Geometry check sheet. Reference: the model listing, model coordinates, mm. A direction names the side the tool comes from. Give positions to 0.01 mm unless a question says otherwise; leave off trailing zeros. Order: outer loops, then holes, each group sorted by start corner. A loop starts at its lowest first (then second) coordinate and runs counter-clockwise, first axis right, second up. Notation, with made-up numbers: M 75.5,35.5 L 115.5,35.5 A10 cw 115.5,52.5 Z; hole C 45.25,-31 d5. An arc over 180 degrees is marked long. Put each result on its own line as item: value. Start each with the question number.
Q1. Material ranges on L1, parallel to X at y = 65, z = 75; L2, parallel to Y at x = 5, z = 81; L3, parallel to Z at x = 26, y = 53.5, recorded low to high.
Q2. Mould release check, pull along X, two halves, no side actions. Record for faces 5 (the cylindrical face through (46.874, 52.497, 0.275)), 6 (the flat face through (56, 1, 16)), 7 (the flat face through (28, 0, 74)): +X half, -X half, draft (parallel to the pull), parting line (faces both ways), or undercut.
Q3. Section check B-B on y = 73. Record the cut outline in (x, z).
Q4. Access from +Z, -Z, +X, -X, +Y, -Y to the whole of each face (thin tool, end or side, straight path). Record for faces 1 (the flat face through (24.5, 60, 103)), 2 (the flat face through (15.5, 60, 103)), 3 (the flat face through (48, -1, 25)), 4 (the cylindrical face through (46.874, -52.497, -0.275)).
Q5. Go/stop test with flat-tipped pins: pin 1 (5.5 mm diameter, centred on x = 49.5, y = -1, fed in from +Z); pin 2 (9.5 mm diameter, centred on x = 4.5, z = 90, fed in from -Y); pin 3 (1 mm diameter, centred on x = 29.5, y = 56, fed in from -Z). Record where each tip stops, or that it passes through.
Q6. Section check C-C on y = -23.5. Record the cut outline in (x, z), then the cut area to 3 significant figures.
Q7. Section check A-A on x = 46. Record the cut outline in (y, z), then the cut area to 3 significant figures.
Q8. Section check D-D on z = 62.5. Record the cut outline in (x, y), then the cut area to 3 significant figures.
```python
from build123d import *

# Parameters (mm, degrees)
BOSS_EXTRUDE1_DEPTH        = 56
BOSS_EXTRUDE2_DEPTH        = 38
BOSS_EXTRUDE3_START        = -0.322075
BOSS_EXTRUDE3_DEPTH        = 100.322075
SKETCH3_R                  = 20
BOSS_EXTRUDE4_DEPTH        = 40
RIB2_START                 = -4.5
RIB2_DEPTH                 = 9
F_10_0MM_DOWEL_HOLE1_D     = 18
F_10_0MM_DOWEL_HOLE1_DEPTH = 32
F_10_0MM_DOWEL_HOLE1_TIP   = 5.407745571


with BuildPart() as part:
    # Sketch1 → Boss-Extrude1 (new body)
    with BuildSketch(Plane(origin=(0, 0, 0), x_dir=(0, 0, -1), z_dir=(1, 0, 0))):
        with BuildLine():
            Line((-25, -40), (-25, 40))
            ThreePointArc((-25, 40), (0, 65), (25, 40))
            Line((25, 40), (25, -40))
            ThreePointArc((25, -40), (0, -65), (-25, -40))
        make_face()
        with BuildLine():
            Line((-12.5, -40), (-12.5, 40))
            ThreePointArc((-12.5, 40), (0, 52.5), (12.5, 40))
            Line((12.5, 40), (12.5, -40))
            ThreePointArc((12.5, -40), (0, -52.5), (-12.5, -40))
        make_face(mode=Mode.SUBTRACT)
    extrude(amount=BOSS_EXTRUDE1_DEPTH)

    # Sketch1<2> → Boss-Extrude2 (add)
    with BuildSketch(Plane(origin=(0, 0, 0), x_dir=(0, 0, -1), z_dir=(1, 0, 0))):
        with BuildLine():
            Line((12.5, -40), (12.5, 40))
            ThreePointArc((12.5, 40), (0, 52.5), (-12.5, 40))
            Line((-12.5, 40), (-12.5, -40))
            ThreePointArc((-12.5, -40), (0, -52.5), (12.5, -40))
        make_face()
    extrude(amount=BOSS_EXTRUDE2_DEPTH)

    # Sketch2 → Boss-Extrude3 (add)
    with BuildSketch(Plane.XY.offset(25).offset(BOSS_EXTRUDE3_START)):
        Polygon((0, 22), (0, 44), (40, 44), (40, -44), (0, -44), (0, -20.015625235), (12, -20.015625235), (12, -32), (28, -32), (28, 32), (12, 32), (12, 22), align=None)
    extrude(amount=BOSS_EXTRUDE3_DEPTH)

    # Sketch3 → Boss-Extrude4 (add)
    with BuildSketch(Plane(origin=(0, 44, 0), x_dir=(1, 0, 0), z_dir=(0, 1, 0))):
        with Locations(Location((20, -75, 0), (0, 0, 180))):
            Circle(SKETCH3_R)
    extrude(amount=BOSS_EXTRUDE4_DEPTH)

    # Rib2: read off the stored shape, not the designer's step
    # Rib2 outline → Rib2 (add)
    with BuildSketch(Plane(origin=(20, 0, 0), x_dir=(0, 0, -1), z_dir=(1, 0, 0)).offset(RIB2_START)):
        Polygon((-125, 44), (-94.48717527, 44), (-94.48717527, 84), (-95, 84), align=None)
    extrude(amount=RIB2_DEPTH)

    # Ø10.0mm Dowel Hole1
    with Locations(Plane(origin=(20, 84, 75), x_dir=(1, 0, 0), z_dir=(0, 1, 0))):
        with Locations((0, 0)):
            Hole(F_10_0MM_DOWEL_HOLE1_D / 2, depth=F_10_0MM_DOWEL_HOLE1_DEPTH)
            with Locations((0, 0, -(F_10_0MM_DOWEL_HOLE1_DEPTH + F_10_0MM_DOWEL_HOLE1_TIP / 2))):  # 118° drill point
                Cone(0, F_10_0MM_DOWEL_HOLE1_D / 2, F_10_0MM_DOWEL_HOLE1_TIP, mode=Mode.SUBTRACT)


solid = part.part
```
Results found:
1. L1: x = 0 to 11, 29 to 40
1. L2: y = -44 to -20.02, 22 to 84
1. L3: z = -21.04 to 21.04, 55.92 to 68.29, 81.71 to 94.08
2. face 5: draft
2. face 6: +X half
2. face 7: undercut
3. outline: M 15.5,94.49 A20 ccw long 24.5,94.49 L 24.5,103.25 L 15.5,103.25 Z; hole C 20,75 d18
4. face 1: +Z, +X, +Y
4. face 2: +Z, -X, +Y
4. face 3: +Z, +X, +Y, -Y
4. face 4: +X
5. pin 1: stops at z = 25
5. pin 2: stops at y = -44
5. pin 3: stops at z = -19.62
6. outline: M 0,-25 L 56,-25 L 56,-12.5 L 38,-12.5 L 38,12.5 L 56,12.5 L 56,25 L 40,25 L 40,125 L 28,125 L 28,25 L 12,25 L 12,125 L 0,125 Z
6. area: 4,750 mm^2
7. outline: M -40,-25 L 40,-25 A25 ccw 40,25 L -40,25 A25 ccw Z; hole M -40,-12.5 L 40,-12.5 A12.5 ccw 40,12.5 L -40,12.5 A12.5 ccw Z
7. area: 3,470 mm^2
8. outline: M 0,-44 L 40,-44 L 40,44 L 35.61,44 L 35.61,84 L 4.39,84 L 4.39,44 L 0,44 L 0,22 L 12,22 L 12,32 L 28,32 L 28,-32 L 12,-32 L 12,-20.02 L 0,-20.02 Z
8. area: 3,240 mm^2
